The model under review builds one solid part; all positions refer to its coordinate system, in mm. Give positions to 0.01 mm unless a question says otherwise; leave off trailing zeros. Loops run counter-clockwise (first coordinate to the right, second up) from the corner with the lowest first, then second, coordinate; pieces in that order, holes last. Notation, with made-up numbers: M -36.5,-17.5 L -21.5,-17.5 A13 cw -21.5,1.5 Z; hole C 59.25,54 d2. An arc over 180 degrees is marked long. Return JSON: item names as keys, results as strings. Group by question number.
Autodesk Inventor part; units mm, degrees
ref_plane "YZ Plane" through (0, 0, 0) normal (1, 0, 0) x (0, 1, 0)
ref_plane "XZ Plane" through (0, 0, 0) normal (0, 1, 0) x (-1, 0, 0)
ref_plane "XY Plane" through (0, 0, 0) normal (0, 0, 1) x (1, 0, 0)
sketch "Sketch1" plane through (0, 0, 0) normal (0, 0, 1) x (1, 0, 0)
  line L0 (-117, -89.5) -> (117, -89.5)
  line L1 (117, -89.5) -> (117, 89.5)
  line L2 (117, 89.5) -> (-117, 89.5)
  line L3 (-117, 89.5) -> (-117, -89.5)
  line L4 (-117, -89.5) -> (117, 89.5) construction
  line L5 (117, -89.5) -> (-117, 89.5) construction
  point P0 (0, 0)
  dimension "d0" = 234
  dimension "d1" = 179
extrude "Extrusion1" add sketch "Sketch1" along normal blind 3
fillet "Fillet1" radius 8 4 edges at (117, -89.5, 1.5) (-117, -89.5, 1.5) (-117, 89.5, 1.5) (117, 89.5, 1.5)
sketch "Sketch2" plane through (0, 0, 3) normal (0, 0, 1) x (1, 0, 0)
  line L0 (-109, -89.5) -> (109, -89.5) construction
  arc A0 (-117, -81.5) -> (-109, -89.5) centre (-109, -81.5) ccw
  line L1 (-117, 81.5) -> (-117, -81.5)
  arc A1 (-109, 89.5) -> (-117, 81.5) centre (-109, 81.5) ccw
  line L2 (109, 89.5) -> (-109, 89.5)
  arc A2 (117, 81.5) -> (109, 89.5) centre (109, 81.5) ccw
  line L3 (117, -81.5) -> (117, 81.5) construction
  arc A3 (109, -89.5) -> (117, -81.5) centre (109, -81.5) ccw construction
  line L4 (-109, -89.5) -> (109, -89.5)
  circle A4 centre (55.5, -89.5) radius 5
  line L5 (117, -81.5) -> (117, 81.5)
  circle A5 centre (117, -39.5) radius 5
  line L6 (-170.275, 0) -> (170.275, 0)
  line L7 (0, 131.775) -> (0, -131.775)
  arc A6 (-117, -81.5) -> (-109, -89.5) centre (-109, -81.5) ccw construction
  circle A7 centre (-55.5, -89.5) radius 5
  circle A8 centre (-117, -39.5) radius 5
  line L8 (-109, 89.5) -> (109, 89.5) construction
  arc A9 (-109, 89.5) -> (-117, 81.5) centre (-109, 81.5) ccw
  arc A10 (117, 81.5) -> (109, 89.5) centre (109, 81.5) ccw construction
  line L9 (-109, 89.5) -> (109, 89.5)
  circle A11 centre (55.5, 89.5) radius 5
  circle A12 centre (117, 39.5) radius 5
  circle A13 centre (-117, 39.5) radius 5
  arc A14 (-109, 89.5) -> (-117, 81.5) centre (-109, 81.5) ccw construction
  circle A15 centre (-55.5, 89.5) radius 5
  point P0 (0, 0)
  point P1 (-50.5, -89.5)
  point P2 (-60.5, -89.5)
  point P3 (-117, -34.5)
  point P4 (-117, -44.5)
  point P5 (-117, 44.5)
  point P6 (-117, 34.5)
  point P7 (-60.5, 89.5)
  point P8 (-50.5, 89.5)
  point P9 (50.5, 89.5)
  point P10 (60.5, 89.5)
  point P11 (117, 44.5)
  point P12 (117, 34.5)
  point P13 (117, -34.5)
  point P14 (117, -44.5)
  point P15 (60.5, -89.5)
  point P16 (50.5, -89.5)
  dimension "d5" = 10
  dimension "d6" = 10
  dimension "d7" = 61.5
  dimension "d8" = 50
extrude "Extrusion2" cut sketch "Sketch2" against normal through all contours L5 A5 | A4 L4 | L1 A8 | A7 L4 | L1 A13 | A12 L5 | L2 A11 | A15 L2 picked at (116.6011, -41.1182) picked at (57.1182, -89.1011) picked at (-115.906, -37.9566) picked at (-53.8818, -89.1011) picked at (-115.906, 41.0434) picked at (115.4959, 40.7959) picked at (57.0242, 88.3266) picked at (-53.9758, 88.3266)
sketch "Sketch3" plane through (0, 0, 3) normal (0, 0, 1) x (1, 0, 0)
  circle A0 centre (104.5, -77.5) radius 1.75
  line L0 (117, -34.5) -> (117, 34.5)
  line L1 (60.5, -89.5) -> (109, -89.5) construction
  line L2 (0, 127.7397) -> (0, -127.7397)
  line L3 (-166.2397, 0) -> (166.2397, 0)
  circle A1 centre (-104.5, -77.5) radius 1.75
  circle A2 centre (104.5, 77.5) radius 1.75
  line L4 (60.5, 89.5) -> (109, 89.5) construction
  circle A3 centre (-104.5, 77.5) radius 1.75
  point P0 (0, 0)
  point P1 (-109, -89.5)
  point P2 (-109, 89.5)
  dimension "d11" = 3.5
  dimension "d33" = 209
  dimension "d34" = 155
extrude "Extrusion3" cut sketch "Sketch3" against normal blind 10
sketch "Sketch4" plane through (0, 0, 3) normal (0, 0, 1) x (1, 0, 0)
  circle A0 centre (-81, -60.5) radius 8
  circle A1 centre (-75, -78.5) radius 2
  line L0 (-33, -78.5) -> (-65, -78.5) construction
  line L1 (-33, -76) -> (-65, -76)
  line L2 (-65, -81) -> (-33, -81)
  arc A2 (-33, -81) -> (-33, -76) centre (-33, -78.5) ccw
  arc A3 (-65, -76) -> (-65, -81) centre (-65, -78.5) ccw
  circle A4 centre (-85, -79.5) radius 1.5
  line L3 (-12.5, -60.5) -> (-95.5, -60.5) construction
  line L4 (-41, -83.5) -> (-41, -33.5) construction
  circle A5 centre (3, -79.5) radius 1.5
  circle A6 centre (-85, -41.5) radius 1.5
  circle A7 centre (3, -41.5) radius 1.5
  line L5 (-109, -89.5) -> (-60.5, -89.5)
  line L6 (-117, -44.5) -> (-117, -81.5)
  point P0 (0, 0)
  point P1 (-49, -78.5)
  dimension "d16" = 2.5
  dimension "d17" = 16
  dimension "d18" = 4
  dimension "d19" = 10
  dimension "d20" = 32
  dimension "d21" = 6
  dimension "d22" = 18
  dimension "d23" = 34
  dimension "d24" = 18
  dimension "d25" = 44
  dimension "d26" = 19
  dimension "d27" = 3
  dimension "d28" = 10
  dimension "d29" = 32
  dimension "d30" = 0
extrude "Extrusion4" cut sketch "Sketch4" against normal through all
sketch "Sketch5" plane through (0, 0, 3) normal (0, 0, 1) x (1, 0, 0)
  circle A0 centre (-81, -60.5) radius 8
  line L0 (-33, -81) -> (-65, -81)
  arc A1 (-65, -76) -> (-65, -81) centre (-65, -78.5) ccw
  line L1 (-65, -76) -> (-33, -76)
  arc A2 (-33, -81) -> (-33, -76) centre (-33, -78.5) ccw
  circle A3 centre (-85, -41.5) radius 1.5
  circle A4 centre (3, -41.5) radius 1.5
  circle A5 centre (-75, -78.5) radius 2
  circle A6 centre (-85, -79.5) radius 1.5
  circle A7 centre (3, -79.5) radius 1.5
  circle A8 centre (-104.5, 77.5) radius 1.75
  circle A9 centre (-104.5, -77.5) radius 1.75
  circle A10 centre (104.5, 77.5) radius 1.75
  circle A11 centre (104.5, -77.5) radius 1.75
  arc A12 (117, 44.5) -> (117, 34.5) centre (117, 39.5) ccw
  line L2 (117, 44.5) -> (117, 81.5)
  arc A13 (117, 81.5) -> (109, 89.5) centre (109, 81.5) ccw
  line L3 (109, 89.5) -> (60.5, 89.5)
  arc A14 (50.5, 89.5) -> (60.5, 89.5) centre (55.5, 89.5) ccw
  line L4 (50.5, 89.5) -> (-50.5, 89.5)
  arc A15 (-60.5, 89.5) -> (-50.5, 89.5) centre (-55.5, 89.5) ccw
  line L5 (-60.5, 89.5) -> (-109, 89.5)
  arc A16 (-109, 89.5) -> (-117, 81.5) centre (-109, 81.5) ccw
  line L6 (-117, 81.5) -> (-117, 44.5)
  arc A17 (-117, 34.5) -> (-117, 44.5) centre (-117, 39.5) ccw
  line L7 (-117, 34.5) -> (-117, -34.5)
  arc A18 (-117, -44.5) -> (-117, -34.5) centre (-117, -39.5) ccw
  line L8 (-117, -44.5) -> (-117, -81.5)
  arc A19 (-117, -81.5) -> (-109, -89.5) centre (-109, -81.5) ccw
  line L9 (-109, -89.5) -> (-60.5, -89.5)
  arc A20 (-50.5, -89.5) -> (-60.5, -89.5) centre (-55.5, -89.5) ccw
  line L10 (-50.5, -89.5) -> (50.5, -89.5)
  arc A21 (60.5, -89.5) -> (50.5, -89.5) centre (55.5, -89.5) ccw
  line L11 (60.5, -89.5) -> (109, -89.5)
  arc A22 (109, -89.5) -> (117, -81.5) centre (109, -81.5) ccw
  line L12 (117, -81.5) -> (117, -44.5)
  arc A23 (117, -34.5) -> (117, -44.5) centre (117, -39.5) ccw
  line L13 (117, -34.5) -> (117, 34.5)
  point P0 (0, 0)
equation "\"d6\" = d5"
properties part number "AcrylicCover"
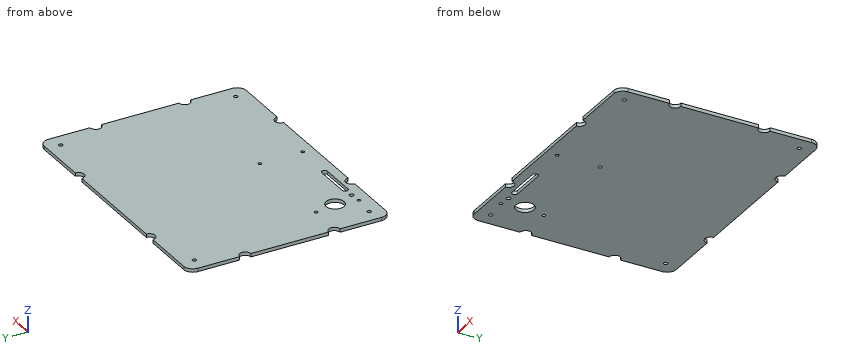
(1) Add section A-A (y = -60.5). Write out the cut boundary in (x, z).
(2) Add section B-B (x = -81). Write out the cut boundary in (y, z).
(3) For pin 1 (0.9 mm diameter, centred on x = -56, z = 1.5, fed in from -Y); pin 2 (3 mm diameter, centred on x = -104.5, y = 77.5, fed in from +Z), all flat-tipped, find the tip position at first contact; note any pin that passes through.
(4) Add section C-C (x = 55.5). Write out the cut boundary in (y, z), and give its area (3 significant figures).
(5) For probe 1 along Y at (x, z) = (-104.5, 1.05); probe 2 along X at (y, z) = (77.5, 1.4); probe 3 along Y at (x, z) = (3, 1.9), list the stretches that pass through material, from the lowest coordinate up.
(6) Add section D-D (z = 0.7). Count the separate pieces of the cut face and the enclosed holes in it, and give its area (3 significant figures).
Verdict:
{
 "1": {"outline": "M -117,0 L -89,0 L -89,3 L -117,3 Z; M -73,0 L 117,0 L 117,3 L -73,3 Z"},
 "2": {"outline": "M -89.5,0 L -68.5,0 L -68.5,3 L -89.5,3 Z; M -52.5,0 L 89.5,0 L 89.5,3 L -52.5,3 Z"},
 "3": {"pin 1": "stops at y = -84.59", "pin 2": "passes through"},
 "4": {"outline": "M -84.5,0 L 84.5,0 L 84.5,3 L -84.5,3 Z", "area": "507 mm²"},
 "5": {"probe 1": "y = -89.5 to -79.25, -75.75 to 75.75, 79.25 to 89.5", "probe 2": "x = -117 to -106.25, -102.75 to 102.75, 106.25 to 117", "probe 3": "y = -89.5 to -81, -78 to -43, -40 to 89.5"},
 "6": {"separate pieces": "1", "enclosed holes": "11", "area": "41,100 mm²"}
}
